Input: part model. Units: mm. Frame: model coordinates. A direction names the side the tool comes from. Give positions to 0.01 mm unless a question says otherwise; leave off trailing zeros. Loops run counter-clockwise (first coordinate to the right, second up) from the corner with the lowest first, then second, coordinate; pieces in that order, holes last. Notation, with made-up numbers: M -33,-24.75 L 5,-24.75 A30 cw 5,0.25 Z; hole C -13.75,-17 d6. An arc over 180 degrees is marked long. Use CSV: the item, a comma, the result in double quotes. Start each with the question number.
from build123d import *

# Parameters (mm, degrees)
SKETCH1_R           = 40
SKETCH1_R_2         = 5
SKETCH1_R_3         = 1
BOSS_EXTRUDE1_DEPTH = 2
CUT_EXTRUDE1_REACH  = 58.604
SKETCH6_R           = 6
BOSS_EXTRUDE4_DEPTH = 13
SKETCH9_R           = 41
CUT_EXTRUDE2_DEPTH  = 11
CUT_EXTRUDE3_DEPTH  = 3
CHAMFER1_SIZE       = 2
SKETCH11_R          = 5
BOSS_EXTRUDE5_DEPTH = 2


with BuildPart() as part:
    # Sketch1 → Boss-Extrude1 (new body)
    with BuildSketch(Plane(origin=(0, 0, 0), x_dir=(1, 0, 0), z_dir=(0, 1, 0))):
        with Locations(Location((0, 0, 0), (0, 0, 270))):
            Circle(SKETCH1_R)
        with Locations(Location((0, 0, 0), (0, 0, 270))):
            Circle(SKETCH1_R_2, mode=Mode.SUBTRACT)
        with Locations(Location((0, 25, 0), (0, 0, 270))):
            Circle(SKETCH1_R_3, mode=Mode.SUBTRACT)
        with Locations(Location((21.650635095, -12.5, 0), (0, 0, 270))):
            Circle(SKETCH1_R_3, mode=Mode.SUBTRACT)
        with Locations(Location((-21.650635095, -12.5, 0), (0, 0, 270))):
            Circle(SKETCH1_R_3, mode=Mode.SUBTRACT)
    extrude(amount=BOSS_EXTRUDE1_DEPTH)

    # Sketch2 → Cut-Extrude1 (cut, up to next)
    with BuildSketch(Plane(origin=(0, 2, 0), x_dir=(1, 0, 0), z_dir=(0, 1, 0)), mode=Mode.PRIVATE) as cut_extrude1_sk1:
        with BuildLine():
            Line((-1, 35), (1, 35))
            ThreePointArc((1, 35), (1.707106781, 35.292893219), (2, 36))
            Line((2, 36), (2, 38))
            ThreePointArc((2, 38), (1.707106781, 38.707106781), (1, 39))
            Line((1, 39), (-1, 39))
            ThreePointArc((-1, 39), (-1.707106781, 38.707106781), (-2, 38))
            Line((-2, 38), (-2, 36))
            ThreePointArc((-2, 36), (-1.707106781, 35.292893219), (-1, 35))
        make_face()
    cut_extrude1_tool1 = extrude(cut_extrude1_sk1.sketch, amount=-CUT_EXTRUDE1_REACH, mode=Mode.PRIVATE) & part.part
    add(cut_extrude1_tool1.solids().sort_by_distance((0, 2, -37))[0], mode=Mode.SUBTRACT)

    # Sketch6 → Boss-Extrude4 (add)
    with BuildSketch(Plane.XZ):
        with Locations(Location((13.680805733, 37.587704831, 0), (0, 0, 270))):
            Circle(SKETCH6_R)
        with Locations(Location((40, 0, 0), (0, 0, 270))):
            Circle(SKETCH6_R)
    boss_extrude4 = extrude(amount=-BOSS_EXTRUDE4_DEPTH)

    # Sketch9 → Cut-Extrude2 (cut)
    with BuildSketch(Plane(origin=(0, 13, 0), x_dir=(1, 0, 0), z_dir=(0, 1, 0))):
        Circle(SKETCH9_R)
    cut_extrude2 = extrude(amount=-CUT_EXTRUDE2_DEPTH, mode=Mode.SUBTRACT)

    # Sketch10 → Cut-Extrude3 (cut)
    with BuildSketch(Plane(origin=(0, 13, 0), x_dir=(1, 0, 0), z_dir=(0, 1, 0))):
        with BuildLine():
            Line((40.972551788, 1.5), (45.809475019, 1.5))
            ThreePointArc((45.809475019, 1.5), (46, 0), (45.809475019, -1.5))
            Line((45.809475019, -1.5), (40.972551788, -1.5))
            ThreePointArc((40.972551788, -1.5), (41, 0), (40.972551788, 1.5))
        make_face()
        with BuildLine():
            Line((15.422976966, -37.988574355), (17.077302143, -42.533795423))
            ThreePointArc((17.077302143, -42.533795423), (15.732926593, -43.225860556), (14.258224281, -43.559855853))
            Line((14.258224281, -43.559855853), (12.603899104, -39.014634785))
            ThreePointArc((12.603899104, -39.014634785), (14.022825876, -38.527397452), (15.422976966, -37.988574355))
        make_face()
    cut_extrude3 = extrude(amount=-CUT_EXTRUDE3_DEPTH, mode=Mode.SUBTRACT)

    # Mirror2: Boss-Extrude4, Cut-Extrude2, Cut-Extrude3 across plane
    add(boss_extrude4.mirror(Plane(origin=(0, 0, 0), x_dir=(0, 0, 1), z_dir=(1, 0, 0))))
    add(cut_extrude2.mirror(Plane(origin=(0, 0, 0), x_dir=(0, 0, 1), z_dir=(1, 0, 0))), mode=Mode.SUBTRACT)
    add(cut_extrude3.mirror(Plane(origin=(0, 0, 0), x_dir=(0, 0, 1), z_dir=(1, 0, 0))), mode=Mode.SUBTRACT)

    # Chamfer1
    chamfer1_edges = [part.edges().sort_by_distance(p)[0] for p in [
        (21.650635095, 2, 11.5),
        (-21.650635095, 2, 11.5),
        (0, 2, -26),
    ]]
    chamfer(chamfer1_edges, length=CHAMFER1_SIZE - 0.0001)  # a hair under: the kernel refuses the full size

    # Sketch11 → Boss-Extrude5 (add)
    with BuildSketch(Plane.XZ):
        with Locations((0, 40)):
            Circle(SKETCH11_R)
        with Locations((16.90473047, -36.252311481)):
            Circle(SKETCH11_R)
        with Locations((-16.90473047, -36.252311481)):
            Circle(SKETCH11_R)
    extrude(amount=-BOSS_EXTRUDE5_DEPTH)


solid = part.part
Item 1: Mould query, pull axis Z, two halves, no side actions, for faces 5 (the flat face through (44, 10, 0)), 6 (the cylindrical face through (46, 6, 0)), 7 (the cylindrical face through (13.944, 7.577, 38.556)), 8 (the flat face through (-43, 13, -3)). Classes: +Z half, -Z half, draft (parallel to the pull), parting line (faces both ways), or undercut.
Item 2: Material intervals for line 1 (X direction, y = 0.05, z = 12.5); line 2 (Y direction, x = 22, z = -31); line 3 (X direction, y = 12, z = 4), sorted ascending.
Item 3: Section B-B (z = 24.5). Output: boundary loops of the cut face in (x, y).
Item 4: First-contact query: pin 1 Ø1.5 at (x, y) = (-44.5, 11) entering from -Z; pin 2 Ø10 at (x, z) = (19.5, -2) entering from +Y; pin 3 Ø1.3 at (x, z) = (15, 39.5) entering from +Y. Flat tips, straight axial feed; report the tip coordinate or a pass-through.
Item 5: Section A-A (y = 4.25). Output: boundary loops of the cut face in (x, z).
Item 6: Section C-C (x = 26). Output: boundary loops of the cut face in (y, z), then the cut area to 3 significant figures.
Item 7: Set-up query: faces 1 (the flat face through (-2, 1, -37)), 2 (the cylindrical face through (6.43, 0.99, 39.48)), 3 (the flat face through (43, 12, -1.5)), 4 (the cylindrical face through (-13.944, 7.577, 38.556)). Return all of +Z, -Z, +X, -X, +Y, -Y with unobstructed straight access to the full face (end or side cutting, diameter ignored); none if empty.
Recorded:
1,face 5,"undercut"
1,face 6,"parting line"
1,face 7,"-Z half"
1,face 8,"draft"
2,line 1,"-38 to -22.7, -20.6 to 20.6, 22.7 to 38"
2,line 2,"0 to 2"
2,line 3,"-44.47 to -40.8, 40.8 to 44.47"
3,outline,"M -31.62,0 L 31.62,0 L 31.62,2 L -31.62,2 Z"
4,pin 1,"z = -4.68"
4,pin 2,"y = 2"
4,pin 3,"y = 10"
5,outline,"M -40.56,-5.97 A41 cw -40.56,5.97 A6 ccw Z; M -19.49,36.07 A41 cw -8.26,40.16 A6 ccw Z; M 8.26,40.16 A41 cw 19.49,36.07 A6 ccw Z; M 40.56,-5.97 A6 ccw 40.56,5.97 A41 cw Z"
6,outline,"M 0,-30.4 L 2,-30.4 L 2,30.4 L 0,30.4 Z"
6,area,"122 mm²"
7,face 1,"+Y, -Y"
7,face 2,"+Z, +Y, -Y"
7,face 3,"+X, -X, +Y"
7,face 4,"-Z, +Y"
